Drawing for the job (mm, zero at the part's lowest x, y, z). Give positions to 0.01 mm unless a question says otherwise; leave off trailing zeros. Loops run counter-clockwise (first coordinate to the right, second up) from the corner with the lowest first, then second, coordinate; pieces in that order, holes last. Notation, with made-up numbers: (-16.5, 86) -> (42.5, 86) arc R6 ccw to (42.5, 93) -> close; hole circle Ø1 at (51, 76.25). An arc over 180 degrees is marked (long way). Write item = value, one per line.
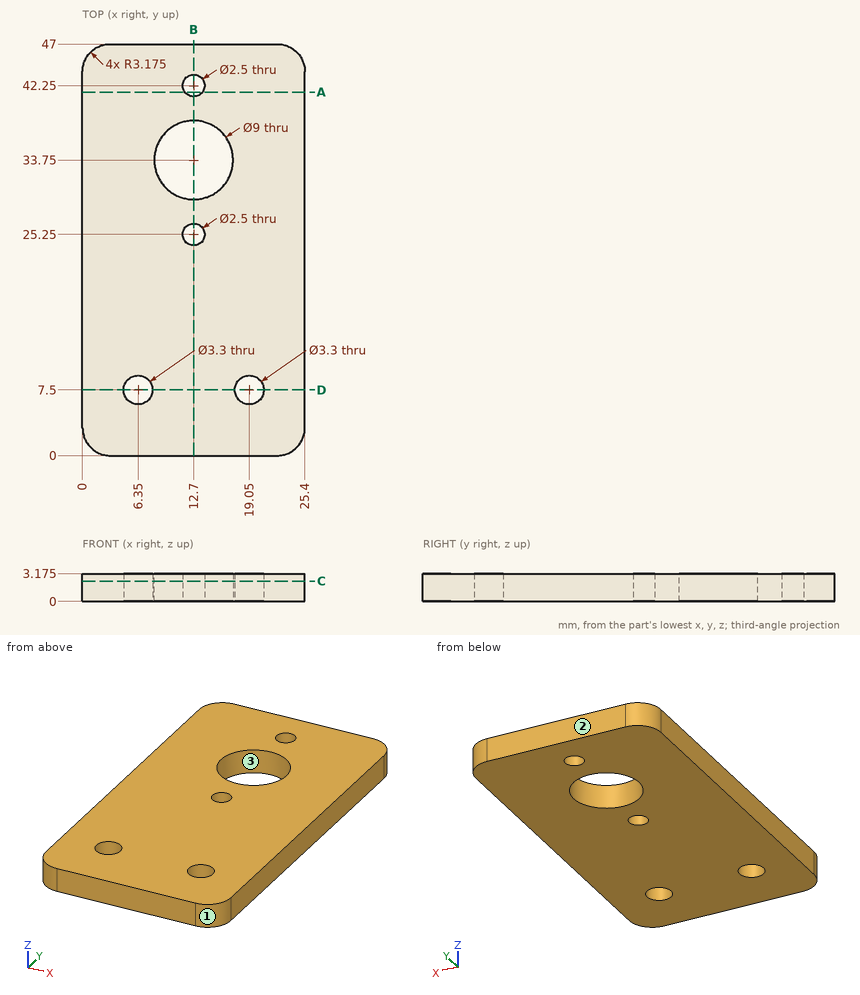
1) Drill centre lines: line 1 along Y through (x, z) = (12.75, 0.5); line 2 along X through (y, z) = (8.5, 1.4); line 3 along Y through (x, z) = (6.25, 0.6). Where is each one in solid material? Low to high. Write a range as [from, to].
Resolved:
line_1 = [0, 24], [26.5, 29.25], [38.25, 41], [43.5, 47]
line_2 = [0, 5.04], [7.66, 17.74], [20.36, 25.4]
line_3 = [0, 5.85], [9.15, 47]
2) Pull direction Y, two halves, no side cores. Call the marked faces 1, 2 and 3: pulls with the +Y half, pulls with the -Y half, needs draft (parallel to the pull), parting line crosses it, or undercut.
Resolved:
face_1 = pulls with the -Y half
face_2 = pulls with the +Y half
face_3 = undercut
3) Slice it at D-D, the plane y = 7.5. List the corners of the cut face in (x, z) (3 decimals).
Resolved:
outline = (0, 0) -> (4.7, 0) -> (4.7, 3.175) -> (0, 3.175) -> close; (8, 0) -> (17.4, 0) -> (17.4, 3.175) -> (8, 3.175) -> close; (20.7, 0) -> (25.4, 0) -> (25.4, 3.175) -> (20.7, 3.175) -> close
4) Slice it at B-B, the plane x = 12.7. List the corners of the cut face in (y, z) (3 decimals), and give its area (3 significant figures).
Resolved:
outline = (0, 0) -> (24, 0) -> (24, 3.175) -> (0, 3.175) -> close; (26.5, 0) -> (29.25, 0) -> (29.25, 3.175) -> (26.5, 3.175) -> close; (38.25, 0) -> (41, 0) -> (41, 3.175) -> (38.25, 3.175) -> close; (43.5, 0) -> (47, 0) -> (47, 3.175) -> (43.5, 3.175) -> close
area = 105 mm²
5) Slice it at A-A, the plane y = 41.5. List the corners of the cut face in (x, z) (3 decimals), and give its area (3 significant figures).
Resolved:
outline = (0, 0) -> (11.7, 0) -> (11.7, 3.175) -> (0, 3.175) -> close; (13.7, 0) -> (25.4, 0) -> (25.4, 3.175) -> (13.7, 3.175) -> close
area = 74.3 mm²
6) Slice it at C-C, the plane z = 2.3. List the corners of the cut face in (x, y) (3 decimals), and give its area (3 significant figures).
Resolved:
outline = (0, 3.175) arc R3.175 ccw to (3.175, 0) -> (22.225, 0) arc R3.175 ccw to (25.4, 3.175) -> (25.4, 43.825) arc R3.175 ccw to (22.225, 47) -> (3.175, 47) arc R3.175 ccw to (0, 43.825) -> close; hole circle Ø3.3 at (6.35, 7.5); hole circle Ø9 at (12.7, 33.75); hole circle Ø2.5 at (12.7, 25.25); hole circle Ø2.5 at (12.7, 42.25); hole circle Ø3.3 at (19.05, 7.5)
area = 1,090 mm²
